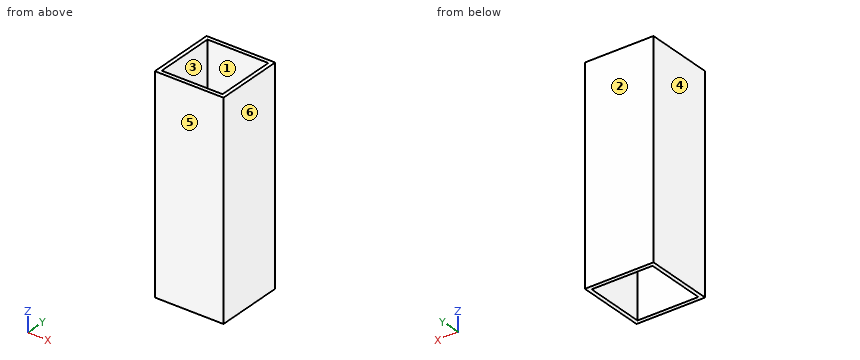
Autodesk Inventor part; units mm, degrees
ref_plane "YZ Plane" through (0, 0, 0) normal (1, 0, 0) x (0, 1, 0)
ref_plane "XZ Plane" through (0, 0, 0) normal (0, 1, 0) x (-1, 0, 0)
ref_plane "XY Plane" through (0, 0, 0) normal (0, 0, 1) x (1, 0, 0)
sketch "Sketch1" plane through (0, 0, 0) normal (0, 0, 1) x (1, 0, 0)
  line L0 (-10.947, -4.6264) -> (19.053, -4.6264)
  line L1 (19.053, -4.6264) -> (19.053, 25.3736)
  line L2 (19.053, 25.3736) -> (-10.947, 25.3736)
  line L3 (-10.947, 25.3736) -> (-10.947, -4.6264)
  line L4 (-10.947, 23.6736) -> (19.053, 23.6736)
  line L5 (-9.247, -4.6264) -> (-9.247, 25.3736)
  line L6 (17.353, -4.6264) -> (17.353, 25.3736)
  line L7 (-10.947, -2.9264) -> (19.053, -2.9264)
  point P0 (0, 0)
  point P1 (-9.247, -2.9264)
  point P2 (17.353, -2.9264)
  point P3 (17.353, 23.6736)
  point P4 (-9.247, 23.6736)
  dimension "d0" = 30
  dimension "d1" = 30
  dimension "d2" = 1.7
  dimension "d3" = 1.7
  dimension "d4" = 1.7
  dimension "d5" = 1.7
extrude "Extrusion1" add sketch "Sketch1" against normal blind 92.042
extrude "Extrusion2" cut sketch "Sketch1" against normal blind 100000 contours L5 L4 L6 L7
properties part number "Cablecanal Ranurado 30x30 L=116 mm" material "PPS Plastic"
For this review, take the finished solid that the model builds, in its own axes (mm). Face numbers are marked on the shaded views. A direction names the side the tool comes from. Round coordinates to 2 decimals unless told otherwise and drop trailing zeros. Write each loop counter-clockwise with the first axis right and the second up, starting at its lowest first coordinate (ties: lowest second). Pieces come first, ordered by that corner, then holes. Notation, with made-up numbers: (40.5, 65.25) - (65.5, 65.25) arc R26 cw to (65.5, 90.25) - close; hole circle Ø6 at (26.25, 45.25). An arc over 180 degrees is marked (long way). Put each result on its own line as item: value.
Q1. We need section B-B (x = 3.5). Give the boundary of the cut face in (y, z).
Solved:
outline: (-4.63, -92.04) - (-2.93, -92.04) - (-2.93, 0) - (-4.63, 0) - close; (23.67, -92.04) - (25.37, -92.04) - (25.37, 0) - (23.67, 0) - close
Q2. Machinability: for the marked faces 1 and 2, which of the approach directions +Z, -Z, +X, -X, +Y, -Y give a long, thin tool a straight path to every point of the face, cutting with its end or side? Answer none if there is none.
Solved:
face 1: +Z, -Z
face 2: +Z, -Z, +X, -X, +Y
Q3. We need section C-C (z = -30.5). Give the boundary of the cut face in (x, y).
Solved:
outline: (-10.95, -4.63) - (19.05, -4.63) - (19.05, 25.37) - (-10.95, 25.37) - close; hole (-9.25, -2.93) - (17.35, -2.93) - (17.35, 23.67) - (-9.25, 23.67) - close
Q4. We need section A-A (y = 6). Give the boundary of the cut face in (x, z), and give its area (3 significant figures).
Solved:
outline: (-10.95, -92.04) - (-9.25, -92.04) - (-9.25, 0) - (-10.95, 0) - close; (17.35, -92.04) - (19.05, -92.04) - (19.05, 0) - (17.35, 0) - close
area: 313 mm2
Q5. Mouldability with a two-part tool opening along X and no side actions: class the marked faces 3, 4, 5 and 6 as released by +X, released by -X, zero draft, split by the parting line, or undercut.
Solved:
face 3: undercut
face 4: released by -X
face 5: zero draft
face 6: released by +X
Q6. Wall thickness on probe 1 along Y at (x, z) = (-9, -21); probe 2 along X at (y, z) = (3.75, -47): over which ranges is each line inside the solid? List them lowest first.
Solved:
probe 1: y = -4.63 to -2.93, 23.67 to 25.37
probe 2: x = -10.95 to -9.25, 17.35 to 19.05
